Check sheet for the modelled part. Datum: model origin and axes. Units: mm. Face numbers are marked on the shaded views. A direction names the side the tool comes from. Round coordinates to 2 decimals unless told otherwise and drop trailing zeros. Order: outer loops, then holes, each group sorted by start corner. A loop starts at its lowest first (then second) coordinate and runs counter-clockwise, first axis right, second up. Notation, with made-up numbers: (-20.5, -17.75) -> (4.5, -17.75) arc R27 ccw to (4.5, 4.25) -> close; hole circle Ø5 at (71, 62.5). An arc over 180 degrees is marked (long way). Answer in a Markdown table with one row per item. Add a question column.
1. Material ranges on L1, parallel to X at y = 0, z = -11; L2, parallel to Y at x = 0, z = 7.75; L3, parallel to Z at x = -3, y = 8.5, recorded low to high. Write a range as from..to.
2. Sectioned sample at A-A, the plane z = 10. Record the boundary of the cut face in (x, y), then the cut area to 3 significant figures.
3. Draft check along X on the marked faces 1, 2 and 3. Enter one of: +X half, -X half, draft (parallel to the pull), parting line (faces both ways), or undercut.
4. Depth check by flat-ended pin: P1, Ø3, axis at x = -10, y = 5, coming from the +Z side; P2, Ø8, axis at x = -4.5, z = 25.5, coming from the -Y side; P3, Ø12, axis at x = -10, z = 31, coming from the +Y side; P4, Ø2, axis at x = 9, y = -3.5, coming from the +Z side. Enter the tip coordinate at first touch or a pass-through.
5. Sectioned sample at B-B, the plane z = 17. Record the boundary of the cut face in (x, y), then the cut area to 3 significant figures.
6. Sectioned sample at C-C, the plane z = -3.5. Record the boundary of the cut face in (x, y).
7. Access from +Z, -Z, +X, -X, +Y, -Y to the whole of each face (thin tool, end or side, straight path). Record for the marked faces 4, 5, 6, 7 and 8.
```python
from build123d import *

# Parameters (mm, degrees)
F0_R      = 15
F1_DEPTH  = 12
F4_R      = 3
F5_DEPTH  = 12
F6_R      = 4.5
F7_DEPTH  = 1.5
F9_DEPTH  = 4
F10_R     = 1.5
F11_DEPTH = 18
F12_R     = 7.5
F13_DEPTH = 10.4
F14_R     = 12.5
F15_DEPTH = 2.4
F16_R     = 5.5
F16_R_2   = 1
F17_DEPTH = 2.4


with BuildPart() as f1:
    # F0 (on Top) → F1 (new body)
    with BuildSketch(Plane.XY):
        Circle(F0_R)
    extrude(amount=F1_DEPTH)

    # F2 (on Front) → F3 (revolve)
    with BuildSketch(Plane.XZ):
        Polygon((11, 14.4), (0, 14.4), (0, 12), (15, 12), (15, 13), align=None)
    revolve(axis=Axis((0, 0, 13.2), (0, 0, -1)))

    # F4 (on face) → F5 (cut)
    with BuildSketch(Plane.XY.offset(14.4)):
        with Locations((0, 9)):
            Circle(F4_R)
        with Locations((-7.794229, 4.5)):
            Circle(F4_R)
        with Locations((-7.794229, -4.5)):
            Circle(F4_R)
        with Locations((0, -9)):
            Circle(F4_R)
        with Locations((7.794229, -4.5)):
            Circle(F4_R)
        with Locations((7.794229, 4.5)):
            Circle(F4_R)
    extrude(amount=-F5_DEPTH, mode=Mode.SUBTRACT)

    # F6 (on face) → F7 (join)
    with BuildSketch(Plane.XY.offset(14.4)):
        Circle(F6_R)
    extrude(amount=F7_DEPTH)

    # F8 (on face) → F9 (join)
    with BuildSketch(Plane.XY.offset(15.9)):
        with BuildLine():
            Line((3.35, -3.00458), (3.35, 3.00458))
            ThreePointArc((3.35, 3.00458), (0, 4.5), (-3.35, 3.00458))
            Line((-3.35, 3.00458), (-3.35, -3.00458))
            ThreePointArc((-3.35, -3.00458), (0, -4.5), (3.35, -3.00458))
        make_face()
    extrude(amount=F9_DEPTH)

    # F10 (on face) → F11 (join)
    with BuildSketch(Plane.XY.offset(19.9)):
        Circle(F10_R)
    extrude(amount=F11_DEPTH)

    # F12 (on face) → F13 (join)
    with BuildSketch(Plane(origin=(0, 0, 0), x_dir=(1, 0, 0), z_dir=(0, 0, -1))):
        Circle(F12_R)
    extrude(amount=F13_DEPTH)

    # F14 (on face) → F15 (join)
    with BuildSketch(Plane(origin=(0, 0, -10.4), x_dir=(1, 0, 0), z_dir=(0, 0, -1))):
        Circle(F14_R)
    extrude(amount=F15_DEPTH)

    # F16 (on face) → F17 (cut)
    with BuildSketch(Plane(origin=(0, 0, -12.8), x_dir=(1, 0, 0), z_dir=(0, 0, -1))):
        Circle(F16_R)
        with Locations((10, 0)):
            Circle(F16_R_2)
        with Locations((-5, 8.660254)):
            Circle(F16_R_2)
        with Locations((-5, -8.660254)):
            Circle(F16_R_2)
    extrude(amount=-F17_DEPTH, mode=Mode.SUBTRACT)


solid = f1.part
```
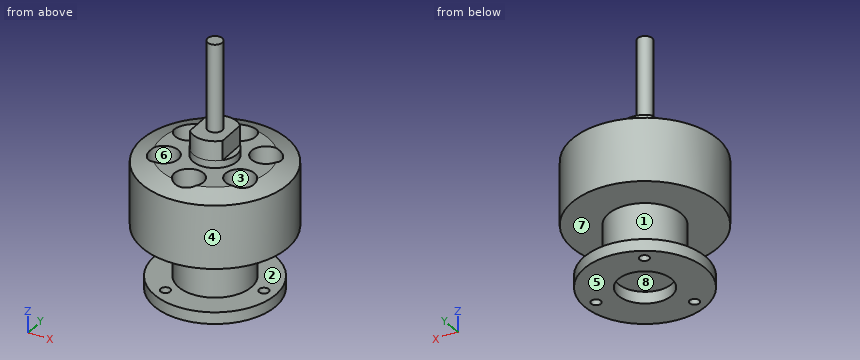
Answer key:
| question | item | result |
|---|---|---|
| 1 | L1 | x = -12.5..-5.5, 5.5..9, 11..12.5 |
| 1 | L2 | y = -15..-12, -6..6, 12..15 |
| 1 | L3 | z = -12.8..-10.4, 0..14.4 |
| 2 | outline | circle Ø30 at (0, 0); hole circle Ø6 at (-7.79, -4.5); hole circle Ø6 at (-7.79, 4.5); hole circle Ø6 at (0, -9); hole circle Ø6 at (0, 9); hole circle Ø6 at (7.79, -4.5); hole circle Ø6 at (7.79, 4.5) |
| 2 | area | 537 mm² |
| 3 | face 1 | parting line |
| 3 | face 2 | draft |
| 3 | face 3 | undercut |
| 4 | P1 | stops at z = 14.3 |
| 4 | P2 | stops at y = -1.41 |
| 4 | P3 | passes through |
| 4 | P4 | stops at z = 2.4 |
| 5 | outline | (-3.35, -3) arc R4.5 ccw to (3.35, -3) -> (3.35, 3) arc R4.5 ccw to (-3.35, 3) -> close |
| 5 | area | 54.1 mm² |
| 6 | outline | circle Ø15 at (0, 0) |
| 7 | face 4 | +Z, -Z |
| 7 | face 5 | -Z, +X, -X, +Y, -Y |
| 7 | face 6 | +Z |
| 7 | face 7 | none |
| 7 | face 8 | -Z |
